Input: part model. Units: mm. Frame: model coordinates. A direction names the side the tool comes from. Coordinates: 2 decimals unless noted, no trailing zeros. Write each loop counter-clockwise with the first axis right and the second up, starting at its lowest first coordinate (ties: lowest second). Pieces come first, ordered by that corner, then holes. Notation, with made-up numbers: M -11.75,-23.5 L 30.25,-23.5 A10 ccw 30.25,-11.5 Z; hole C -36,86.25 d7. An arc over 180 degrees is marked long. Use CSV: the item, a comma, the result in double quotes.
```python
from build123d import *

# Parameters (mm, degrees)
SKETCH_1_W          = 40
SKETCH_1_H          = 78
EXTRUDE_1_DEPTH     = 21.5
SHELL_1_T           = -2
SKETCH_2_R          = 1.6
CUT_EXTRUDE_1_DEPTH = 40


with BuildPart() as part:
    # Эскиз1 → Бобышка-Вытянуть1 (new body)
    with BuildSketch(Plane(origin=(0, 0, 0), x_dir=(1, 0, 0), z_dir=(0, 1, 0))):
        with Locations((20, 39)):
            Rectangle(SKETCH_1_W, SKETCH_1_H)
    extrude(amount=EXTRUDE_1_DEPTH)

    # Оболочка1
    shell_1_openings = [part.faces().sort_by_distance(p)[0] for p in [
        (20, 21.5, -39),
    ]]
    offset(amount=SHELL_1_T, openings=shell_1_openings, kind=Kind.INTERSECTION)

    # Эскиз2 → Вырез-Вытянуть1 (cut)
    with BuildSketch(Plane(origin=(0, 21.5, 0), x_dir=(1, 0, 0), z_dir=(0, 1, 0))):
        with Locations(Location((10.35, 66.81, 0), (0, 0, 90))):
            Circle(SKETCH_2_R)
        with Locations(Location((29.65, 66.81, 0), (0, 0, 90))):
            Circle(SKETCH_2_R)
        with Locations(Location((29.65, 11.19, 0), (0, 0, 90))):
            Circle(SKETCH_2_R)
        with Locations(Location((10.35, 11.19, 0), (0, 0, 90))):
            Circle(SKETCH_2_R)
    extrude(amount=-CUT_EXTRUDE_1_DEPTH, mode=Mode.SUBTRACT)


solid = part.part
```
1. Section B-B (z = -21). Return loops of the section in (x, y).
Resolved:
outline,"M 0,0 L 40,0 L 40,21.5 L 38,21.5 L 38,2 L 2,2 L 2,21.5 L 0,21.5 Z"
2. Section A-A (x = 10.35). Return loops of the section in (y, z), then the cut area to 3 significant figures.
Resolved:
outline,"M 0,-78 L 21.5,-78 L 21.5,-76 L 2,-76 L 2,-68.41 L 0,-68.41 Z; M 0,-65.21 L 2,-65.21 L 2,-12.79 L 0,-12.79 Z; M 0,-9.59 L 2,-9.59 L 2,-2 L 21.5,-2 L 21.5,0 L 0,0 Z"
area,"221 mm^2"
3. Material intervals for line 1 (Z direction, x = 10.35, y = 1.55); line 2 (X direction, y = 0.55, z = -11.19); line 3 (X direction, y = 6.25, z = -47), sorted ascending. Write a range as [from, to].
Resolved:
line 1,"z = [-78, -68.41], [-65.21, -12.79], [-9.59, 0]"
line 2,"x = [0, 8.75], [11.95, 28.05], [31.25, 40]"
line 3,"x = [0, 2], [38, 40]"
4. Section D-D (z = -11.19). Return loops of the section in (x, y), then the cut area to 3 significant figures.
Resolved:
outline,"M 0,0 L 8.75,0 L 8.75,2 L 2,2 L 2,21.5 L 0,21.5 Z; M 11.95,0 L 28.05,0 L 28.05,2 L 11.95,2 Z; M 31.25,0 L 40,0 L 40,21.5 L 38,21.5 L 38,2 L 31.25,2 Z"
area,"145 mm^2"
5. Section C-C (y = 13.5). Return loops of the section in (x, z), then the cut area to 3 significant figures.
Resolved:
outline,"M 0,-78 L 40,-78 L 40,0 L 0,0 Z; hole M 2,-76 L 38,-76 L 38,-2 L 2,-2 Z"
area,"456 mm^2"
6. Contact query for flat-ended pins moving along their axis: pin 1 Ø4 at (x, z) = (29.65, -11.19) entering from +Y; pin 2 Ø10 at (x, z) = (35.5, -45.5) entering from -Y; pin 3 Ø3 at (x, z) = (10.35, -11.19) entering from -Y. Output: stop coordinate, or through.
Resolved:
pin 1,"stops at y = 2"
pin 2,"stops at y = 0"
pin 3,"passes through"
7. Access query for faces 1 (the cylindrical face through (9.869, 1.014, -68.336)), 2 (the flat face through (2, 12, -38)). Directions: +Z, -Z, +X, -X, +Y, -Y. A direction counts if a zero-diameter tool reaches every point of the face in a straight line with its end or side. Return the directions, or none.
Resolved:
face 1,"+Y, -Y"
face 2,"+Y"
8. Mould query, pull axis Z, two halves, no side actions, for faces 3 (the flat face through (20, 11, -78)), 4 (the flat face through (20, 12, -76)), 5 (the flat face through (40, 11, -38)). Classes: pulls with the +Z half, pulls with the -Z half, needs draft (parallel to the pull), parting line crosses it, or undercut.
Resolved:
face 3,"pulls with the -Z half"
face 4,"undercut"
face 5,"needs draft"
